Here's the drawing with two shaded views (mm, measured from the low corner). I have some questions. Round coordinates to 2 decimals unless told otherwise and drop trailing zeros. Loops run counter-clockwise (first coordinate to the right, second up) from the corner with the lowest first, then second, coordinate; pieces in that order, holes last. Notation, with made-up numbers: M 25,87 L 84,87 A22 cw 84,119 Z; hole C 75,40 d1. An arc over 180 degrees is marked long. Answer as a JSON object with one key per item and string values.
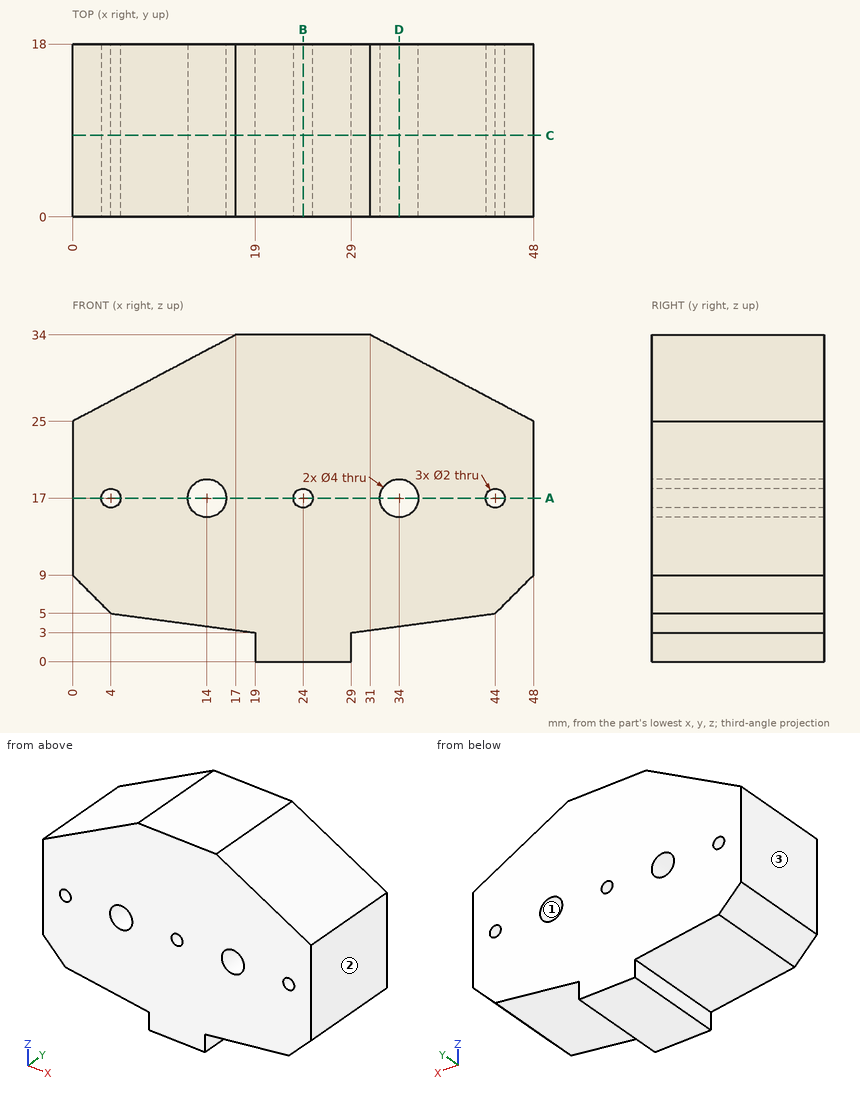
Item 1: I want a section at A-A on z = 17. List the corners of the cut face in (x, y) for me, plus the area to 3 significant figures.
Solution:
{"outline": "M 0,0 L 3,0 L 3,18 L 0,18 Z; M 5,0 L 12,0 L 12,18 L 5,18 Z; M 16,0 L 23,0 L 23,18 L 16,18 Z; M 25,0 L 32,0 L 32,18 L 25,18 Z; M 36,0 L 43,0 L 43,18 L 36,18 Z; M 45,0 L 48,0 L 48,18 L 45,18 Z", "area": "612 mm2"}
Item 2: If I drill on L1, parallel to X at y = 10.5, z = 17; L2, parallel to Z at x = 34, y = 11.25; L3, parallel to Z at x = 44, y = 12, over which ranges is the centre line in solid material (lowest first)? Write a range as from..to.
Solution:
{"L1": "x = 0..3, 5..12, 16..23, 25..32, 36..43, 45..48", "L2": "z = 3.67..15, 19..32.41", "L3": "z = 5..16, 18..27.12"}
Item 3: For P1, Ø5, axis at y = 8.5, z = 6, coming from the -X side; P2, Ø1.2, axis at x = 4, z = 17, coming from the +Y side; P3, Ø4, axis at x = 39.5, y = 6, coming from the +Z side; P4, Ø0.9, axis at y = 8, z = 1, coming from the +X side, each with a flat end and sliding along its axis, tell me the tip position at first contact or that it passes through.
Solution:
{"P1": "stops at x = 0.5", "P2": "passes through", "P3": "stops at z = 30.56", "P4": "stops at x = 29"}
Item 4: I want a section at D-D on x = 34. List the corners of the cut face in (y, z) for me.
Solution:
{"outline": "M 0,3.67 L 18,3.67 L 18,15 L 0,15 Z; M 0,19 L 18,19 L 18,32.41 L 0,32.41 Z"}
Item 5: We'd pull the mould along X, two halves only. Please class the marked faces 1, 2 and 3: +X half, -X half, draft (parallel to the pull), parting line (faces both ways), or undercut.
Solution:
{"face 1": "undercut", "face 2": "+X half", "face 3": "-X half"}
Item 6: I want a section at C-C on y = 8.5. List the corners of the cut face in (x, z) for me, plus the area to 3 significant figures.
Solution:
{"outline": "M 0,9 L 4,5 L 19,3 L 19,0 L 29,0 L 29,3 L 44,5 L 48,9 L 48,25 L 31,34 L 17,34 L 0,25 Z; hole C 4,17 d2; hole C 14,17 d4; hole C 24,17 d2; hole C 34,17 d4; hole C 44,17 d2", "area": "1,270 mm2"}
Item 7: I want a section at B-B on x = 24. List the corners of the cut face in (y, z) for me, plus the area to 3 significant figures.
Solution:
{"outline": "M 0,0 L 18,0 L 18,16 L 0,16 Z; M 0,18 L 18,18 L 18,34 L 0,34 Z", "area": "576 mm2"}
